Print and shaded views of the part. All mm, measured from the part's lowest x, y and z. Give positions to 0.01 mm unless a question says otherwise; leave off trailing zeros. Write each loop counter-clockwise with the first axis right and the second up, starting at its lowest first coordinate (ties: lowest second). Pieces come first, ordered by that corner, then holes. Notation, with made-up numbers: (16, -4.5) - (22, -4.5) arc R15 cw to (22, 10.5) - close; hole circle Ø5 at (33, 50). An arc over 180 degrees is marked (long way). Use one line per item in the form item = value. Start each with the question number.
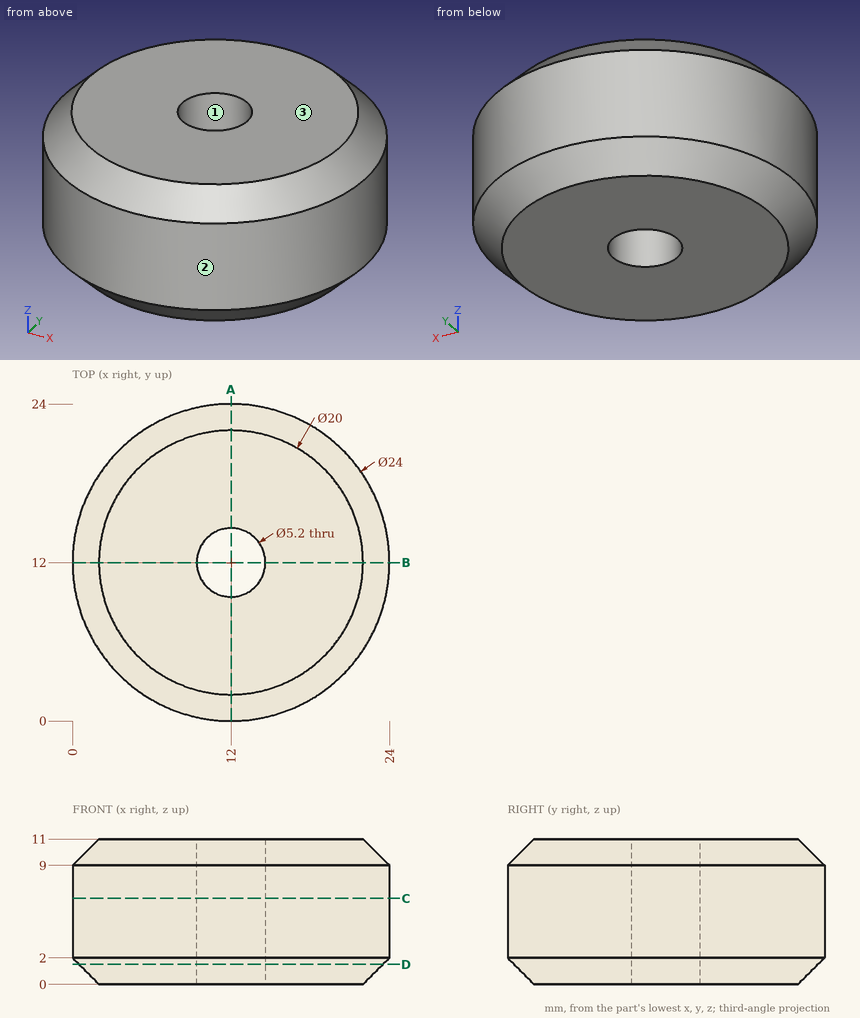
(1) Cut at D-D, the plane z = 1.5. Give the cut face in (x, y), then the cut area to 3 significant figures.
(2) Pin check, flat tips, straight feed: pin 1 Ø1.5 at (y, z) = (14, 6) entering from -X; pin 2 Ø2 at (x, z) = (19, 4) entering from +Y; pin 3 Ø1 at (y, z) = (21.5, 2.5) entering from -X. Stop position of each tip, or through.
(3) Cut at A-A, the plane x = 12. Give the cut face in (y, z), then the cut area to 3 significant figures.
(4) Two-plate mould, pull along Y, no slides. Class the marked faces 1, 2 and 3: +Y half, -Y half, draft (parallel to the pull), parting line (faces both ways), or undercut.
(5) Cut at C-C, the plane z = 6.5. Give the cut face in (x, y), then the cut area to 3 significant figures.
(6) Wall check: line 1 (Y direction, x = 12, z = 4.5); line 2 (X direction, y = 10.25, z = 3.5); line 3 (X direction, y = 9.75, z = 5.5). Give the ranges that are in metal, low to high. Write a range as from..to.
Solution:
q1.outline = circle Ø23 at (12, 12); hole circle Ø5.2 at (12, 12)
q1.area = 394 mm2
q2.pin_1 = 0.07
q2.pin_2 = 22.39
q2.pin_3 = 4.06
q3.outline = (0, 2) - (2, 0) - (9.4, 0) - (9.4, 11) - (2, 11) - (0, 9) - close; (14.6, 0) - (22, 0) - (24, 2) - (24, 9) - (22, 11) - (14.6, 11) - close
q3.area = 199 mm2
q4.face_1 = undercut
q4.face_2 = parting line
q4.face_3 = draft
q5.outline = circle Ø24 at (12, 12); hole circle Ø5.2 at (12, 12)
q5.area = 431 mm2
q6.line_1 = 0..9.4, 14.6..24
q6.line_2 = 0.13..10.08, 13.92..23.87
q6.line_3 = 0.21..10.7, 13.3..23.79
